Source: three-view drawing plus pictorial views. Frame: mm from the lowest corner of the part. Give positions to 0.01 mm unless a question says otherwise; leave off trailing zeros. Loops run counter-clockwise (first coordinate to the right, second up) from the corner with the lowest first, then second, coordinate; pieces in that order, holes last. Notation, with made-up numbers: (0.25, 67.25) - (31.25, 67.25) arc R28 ccw to (31.25, 93.25) - close; hole circle Ø5 at (57, -16.5). An arc over 180 degrees is marked (long way). Answer as a JSON object with one key per item and string values.
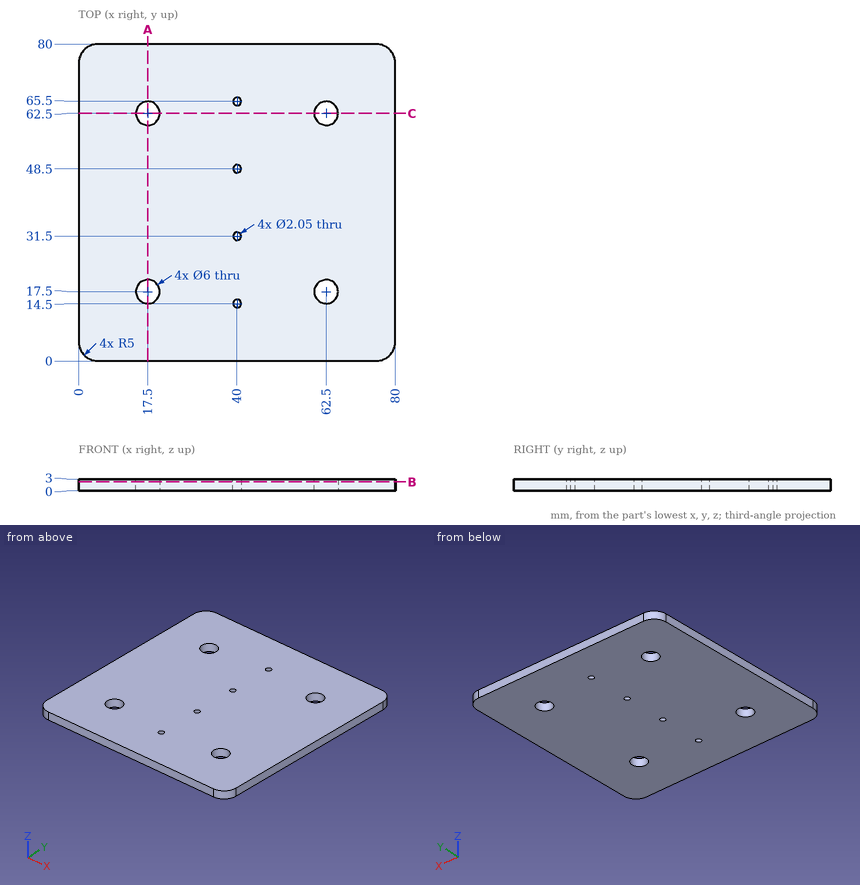
Item 1: Cut plane A-A (x = 17.5). Return loops of the section in (y, z), then the cut area to 3 significant figures.
Geometry check:
{"outline": "(0, 0) - (14.5, 0) - (14.5, 3) - (0, 3) - close; (20.5, 0) - (59.5, 0) - (59.5, 3) - (20.5, 3) - close; (65.5, 0) - (80, 0) - (80, 3) - (65.5, 3) - close", "area": "204 mm2"}
Item 2: Cut plane B-B (z = 2.25). Give the number of separate pieces and of enclosed holes in the cut face, then the cut area to 3 significant figures.
Geometry check:
{"separate pieces": "1", "enclosed holes": "8", "area": "6,250 mm2"}
Item 3: Material intervals for line 1 (Y direction, x = 40, z = 1.5) (3 decimals); line 2 (Y direction, x = 17.5, z = 1.3); line 3 (X direction, y = 17, z = 1.3), sorted ascending. Write a range as [from, to].
Geometry check:
{"line 1": "y = [0, 13.475], [15.525, 30.475], [32.525, 47.475], [49.525, 64.475], [66.525, 80]", "line 2": "y = [0, 14.5], [20.5, 59.5], [65.5, 80]", "line 3": "x = [0, 14.54], [20.46, 59.54], [65.46, 80]"}
Item 4: Contact query for a flat-ended pin moving along its axis: P1, Ø5, axis at x = 62.5, y = 62.5, coming from the -Z side. Output: stop coordinate, or through.
Geometry check:
{"P1": "passes through"}
